```python
from build123d import *

# Parameters (mm, degrees)
F0_R     = 34.925
F1_DEPTH = 38.1
F2_DEPTH = 38.1
F4_DEPTH = 25.4


with BuildPart() as f1:
    # F0 (on Top) → F1 (new body, symmetric)
    with BuildSketch(Plane.XY):
        with BuildLine():
            ThreePointArc((37.567107, -6.35), (37.966543, -3.186161), (38.1, 0))
            ThreePointArc((38.1, 0), (37.966543, 3.186161), (37.567107, 6.35))
            ThreePointArc((37.567107, 6.35), (-38.1, 0), (37.567107, -6.35))
        make_face()
        Circle(F0_R, mode=Mode.SUBTRACT)
    extrude(amount=F1_DEPTH, both=True)

    # F0 (on Top) → F2 (join, symmetric)
    with BuildSketch(Plane.XY):
        with BuildLine():
            ThreePointArc((37.567107, 6.35), (37.966543, 3.186161), (38.1, 0))
            ThreePointArc((38.1, 0), (37.966543, -3.186161), (37.567107, -6.35))
            Line((37.567107, -6.35), (45.374916, -4.865875))
            ThreePointArc((45.374916, -4.865875), (39.497, 0), (45.374916, 4.865875))
            Line((45.374916, 4.865875), (37.567107, 6.35))
        make_face()
        with BuildLine():
            ThreePointArc((49.403, 0), (48.265319, 3.158409), (45.374916, 4.865875))
            ThreePointArc((45.374916, 4.865875), (39.497, 0), (45.374916, -4.865875))
            ThreePointArc((45.374916, -4.865875), (48.265319, -3.158409), (49.403, 0))
        make_face()
    extrude(amount=F2_DEPTH, both=True)

    # F3 (on Top) → F4 (cut)
    with BuildSketch(Plane.XY):
        with BuildLine():
            Line((-42.947944, 0), (39.505817, 0))
            ThreePointArc((39.505817, 0), (41.325165, 3.794629), (45.400634, 4.843333))
            Line((45.400634, 4.843333), (38.253166, 6.174064))
            Line((38.253166, 6.174064), (38.253166, 40.875405))
            Line((38.253166, 40.875405), (-42.947944, 40.875405))
            Line((-42.947944, 40.875405), (-42.947944, 0))
        make_face()
    extrude(amount=-F4_DEPTH, mode=Mode.SUBTRACT)


solid = f1.part
```
Model file for the job. Use its own axes, mm. A direction names the side the tool comes from. Coordinates: 2 decimals unless noted, no trailing zeros. Write each loop counter-clockwise with the first axis right and the second up, starting at its lowest first coordinate (ties: lowest second). Pieces come first, ordered by that corner, then holes. Notation, with made-up numbers: (-1.75, -39.75) - (11.25, -39.75) arc R26 ccw to (11.25, -9.75) - close; hole circle Ø1 at (22.25, 35). An arc over 180 degrees is marked (long way). Use a Markdown table: item, result. Add a question column.
Item 1: Band-saw the part on B-B, the plane y = 8. Write the cut outline in (x, z).
Item 2: Drill centre lines: line 1 along Y through (x, z) = (0, 7) (3 decimals); line 2 along Y through (x, z) = (0, -14.5) (3 decimals); line 3 along X through (y, z) = (-9, 22.5). Where is each one in solid material? Low to high.
Item 3: Two-plate mould, pull along Z, no slides. Class faces 4 (the face through (41.278, 3.756, -12.522)), 5 (the face through (41.526, 5.598, 0.533)), 6 (the face through (35, -5, -38.1)): pulls with the +Z half, pulls with the -Z half, needs draft (parallel to the pull), parting line crosses it, or undercut.
Item 4: Band-saw the part on D-D, the plane y = -12. Write the cut outline in (x, z), and give its area (3 significant figures).
Item 5: Band-saw the part on C-C, the plane z = 18. Write the cut outline in (x, y) (3 decimals), and give its area (3 significant figures).
Item 6: Band-saw the part on A-A, the plane x = 0. Write the cut outline in (y, z) (3 decimals), and give its area (3 significant figures).
Item 7: Drop flat-ended pins along their axis: pin 1 (5 mm diameter, centred on x = 36.5, z = -9, fed in from +Y); pin 2 (8 mm diameter, centred on x = -10.5, z = 19, fed in from +Y); pin 3 (1.5 mm diameter, centred on x = -11, z = -0.5, fed in from -Y). Give the stop position or say it passes through.
Item 8: 3-axis set-ups, long thin cutter, end or side, ignore diameter. For faces 1 (the face through (-37, 0, -13)), 2 (the face through (41.416, -5.618, 0.533)), 3 (the face through (37, 0, -13)): which of +Z, -Z, +X, -X, +Y, -Y reach the whole face in a straight line?
A:
| question | item | result |
|---|---|---|
| 1 | outline | (-37.25, -38.1) - (-34, -38.1) - (-34, -25.4) - (-37.25, -25.4) - close; (-37.25, 0) - (-34, 0) - (-34, 38.1) - (-37.25, 38.1) - close; (34, -38.1) - (37.25, -38.1) - (37.25, -25.4) - (34, -25.4) - close; (34, 0) - (37.25, 0) - (37.25, 38.1) - (34, 38.1) - close |
| 2 | line 1 | y = -38.1 to -34.925, 34.925 to 38.1 |
| 2 | line 2 | y = -38.1 to -34.925 |
| 2 | line 3 | x = -37.02 to -33.75, 33.75 to 37.02 |
| 3 | face 4 | undercut |
| 3 | face 5 | needs draft |
| 3 | face 6 | pulls with the -Z half |
| 4 | outline | (-36.16, -38.1) - (-32.8, -38.1) - (-32.8, 38.1) - (-36.16, 38.1) - close; (32.8, -38.1) - (36.16, -38.1) - (36.16, 38.1) - (32.8, 38.1) - close |
| 4 | area | 512 mm² |
| 5 | outline | (37.567, -6.35) - (45.375, -4.866) arc R4.953 ccw to (49.403, 0) arc R4.953 ccw to (45.375, 4.866) - (37.567, 6.35) arc R38.1 ccw (long way) to start; hole circle Ø69.85 at (0, 0) |
| 5 | area | 841 mm² |
| 6 | outline | (-38.1, -38.1) - (-34.925, -38.1) - (-34.925, 38.1) - (-38.1, 38.1) - close; (34.925, -38.1) - (38.1, -38.1) - (38.1, -25.4) - (34.925, -25.4) - close; (34.925, 0) - (38.1, 0) - (38.1, 38.1) - (34.925, 38.1) - close |
| 6 | area | 403 mm² |
| 7 | pin 1 | stops at y = 6.22 |
| 7 | pin 2 | stops at y = 37.54 |
| 7 | pin 3 | stops at y = -36.7 |
| 8 | face 1 | -X, +Y |
| 8 | face 2 | +Z, -Z, +X, -Y |
| 8 | face 3 | -X |
